Input: part model. Units: mm. Frame: model coordinates. Face numbers are marked on the shaded views. A direction names the side the tool comes from. Round coordinates to 2 decimals unless told otherwise and drop trailing zeros. Loops run counter-clockwise (first coordinate to the right, second up) from the corner with the lowest first, then second, coordinate; pieces in that order, holes last.
(1) Access query for the marked faces 5 and 6. Directions: +Z, -Z, +X, -X, +Y, -Y. A direction counts if a zero-diameter tool reaches every point of the face in a straight line with its end or side. Return the directions, or none.
(2) Draft query along Y for the marked faces 1, 2, 3 and 4. Return one class per face: released by +Y, released by -Y, zero draft, split by the parting line, or undercut.
(3) First-contact query: pin 1 Ø1.5 at (x, y) = (-6.5, 5) entering from +Z. Flat tip, straight axial feed; report the tip coordinate or a pass-through.
(4) Line query: line 1 (X direction, y = 7.75, z = -3); line 2 (Y direction, x = -3.75, z = 6.75); line 3 (X direction, y = 5.25, z = -6). Output: solid intervals per line, ascending.
(5) Cut plane A-A, the plane x = 4. Output: boundary loops of the cut face in (y, z), and give its area (3 significant figures).
(6) Cut plane B-B, the plane y = 5. Output: boundary loops of the cut face in (x, z).
(7) Cut plane D-D, the plane y = 6.75. Output: boundary loops of the cut face in (x, z), and give its area (3 significant figures).
(8) Cut plane C-C, the plane z = -2.75. Output: boundary loops of the cut face in (x, y), and give its area (3 significant figures).
from build123d import *

# Parameters (mm, degrees)
F0_W        = 4
F0_H        = 2
F0_W_2      = 2
F0_H_2      = 4
F0_W_3      = 6.5
F1_DEPTH    = 15
F2_T1_DEPTH = 33


# Not quite as in the source:
# - a fillet or chamfer that OpenCascade refuses, or shapes differently, is made with other operations: its cross-section is extruded or revolved along the edge and cut away or added


with BuildPart() as f1:
    # F0 (on Top) → F1 (new body, symmetric)
    with BuildSketch(Plane.XY):
        with Locations((-4.5, 7)):
            Rectangle(F0_W, F0_H)
        with Locations((-7.5, 7)):
            Rectangle(F0_W_2, F0_H)
        with Locations((-7.5, 4)):
            Rectangle(F0_W_2, F0_H_2)
        with Locations((-7.5, 1)):
            Rectangle(F0_W_2, F0_H)
        with Locations((-3.25, 1)):
            Rectangle(F0_W_3, F0_H)
        with Locations((3.25, 1)):
            Rectangle(F0_W_3, F0_H)
        with Locations((7.5, 1)):
            Rectangle(F0_W_2, F0_H)
        with Locations((7.5, 4)):
            Rectangle(F0_W_2, F0_H_2)
        with Locations((7.5, 7)):
            Rectangle(F0_W_2, F0_H)
        with Locations((4.5, 7)):
            Rectangle(F0_W, F0_H)
    extrude(amount=F1_DEPTH, both=True)

    # F2: fillet of radius 5 on 2 edges, made by hand

    # F2_s2 → F2_t1 (cut)
    with BuildSketch(Plane.XZ.offset(-20.5)):
        with BuildLine():
            ThreePointArc((-8.5, -10), (-7.0355339059, -13.5355339059), (-3.5, -15))
            Line((-3.5, -15), (-8.5, -15))
            Line((-8.5, -15), (-8.5, -10))
        make_face()
        with BuildLine():
            ThreePointArc((-8.5, 10), (-7.0355339059, 13.5355339059), (-3.5, 15))
            Line((-3.5, 15), (-8.5, 15))
            Line((-8.5, 15), (-8.5, 10))
        make_face()
    extrude(amount=F2_T1_DEPTH, mode=Mode.SUBTRACT)


solid = f1.part
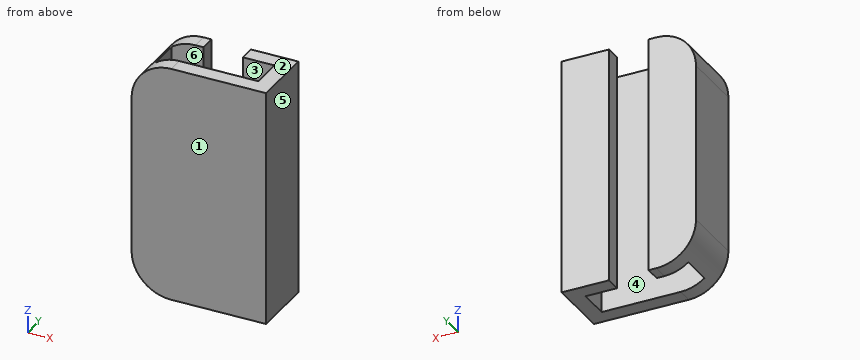
Reported:
1. face 5: +Z, -Z, +X, +Y, -Y
1. face 6: +Z, -Z
2. face 1: released by -Y
2. face 2: zero draft
2. face 3: undercut
2. face 4: undercut
3. pin 1: stops at z = 14
4. line 1: x = -8.5 to -2.5, 2.5 to 8.5
4. line 2: y = 0 to 2, 6 to 8
4. line 3: x = -8.5 to -6.5, 6.5 to 8.5
5. outline: (0, -15) - (2, -15) - (2, 15) - (0, 15) - close; (6, -15) - (8, -15) - (8, 15) - (6, 15) - close
5. area: 120 mm2
6. outline: (-8.5, -10) arc R5 ccw to (-6.5, -14) - (-6.5, 14) arc R5 ccw to (-8.5, 10) - close; (6.5, -15) - (8.5, -15) - (8.5, 15) - (6.5, 15) - close
7. outline: (-8.5, -10) arc R5 ccw to (-3.5, -15) - (-2.5, -15) - (-2.5, 15) - (-3.5, 15) arc R5 ccw to (-8.5, 10) - close; (2.5, -15) - (8.5, -15) - (8.5, 15) - (2.5, 15) - close
7. area: 349 mm2
8. outline: (-8.5, 0) - (8.5, 0) - (8.5, 8) - (2.5, 8) - (2.5, 6) - (6.5, 6) - (6.5, 2) - (-6.5, 2) - (-6.5, 6) - (-2.5, 6) - (-2.5, 8) - (-8.5, 8) - close
8. area: 74.0 mm2
